Autodesk Inventor part; units mm, degrees
ref_plane "YZ Plane" through (0, 0, 0) normal (1, 0, 0) x (0, 1, 0)
ref_plane "XZ Plane" through (0, 0, 0) normal (0, 1, 0) x (-1, 0, 0)
ref_plane "XY Plane" through (0, 0, 0) normal (0, 0, 1) x (1, 0, 0)
sketch "Sketch1" plane through (0, 0, 0) normal (0, 0, 1) x (1, 0, 0)
  line L0 (0, 27.0856) -> (-1.414, 28.5)
  line L1 (-1.414, 28.5) -> (-1.414, 30)
  line L2 (-1.414, 30) -> (1.414, 30)
  line L3 (1.414, 30) -> (1.414, 28.5)
  line L4 (1.414, 28.5) -> (0, 27.0856)
  line L5 (-5, 0) -> (5, 0)
  point P0 (0, 0)
  point P1 (0, 30)
  point P2 (0, 0)
  dimension "d0" = 2
  dimension "d1" = 10
  dimension "d3" = 57
  dimension "d4" = 2.828
  dimension "d5" = 1.5
revolve "Revolution1" add sketch "Sketch1" angle 330 about axis through (-5, 0, 0) along (1, 0, 0)
properties part number "Pierścień klinowy"
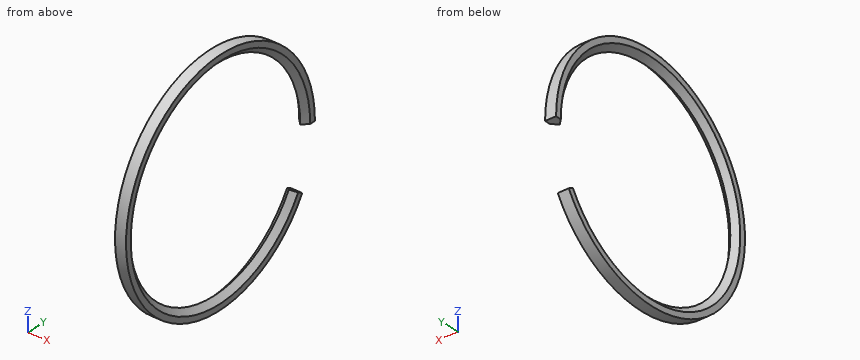
Source: CAD feature listing. Evaluate the final solid. Frame: model axes, mm. Round coordinates to 2 decimals unless told otherwise and drop trailing zeros. Loops run counter-clockwise (first coordinate to the right, second up) from the corner with the lowest first, then second, coordinate; pieces in that order, holes last. Notation, with made-up numbers: (63.25, 25.25) - (115.25, 25.25) arc R22 ccw to (115.25, 63.25) - close; hole circle Ø4 at (18, -26.5). An arc over 180 degrees is marked (long way). Write item = value, one per line. Start each with the question number.
(1) Pin query (flat end, axial travel): pin 1 (1 mm diameter, centred on x = 0, z = 15.5, fed in from -Y); pin 2 (1 mm diameter, centred on x = 1, y = 15.5, fed in from +Z); pin 3 (1.5 mm diameter, centred on x = -1, z = -21.5, fed in from +Y); pin 4 (8 mm diameter, centred on y = -0.5, z = -21.5, fed in from -X). Return the tip coordinate at first contact, or that it passes through.
(2) Ray query, line 1 along Z through (x, y) = (0.2, 1.5); line 2 along Y through (x, z) = (0.95, 10); line 3 along Y through (x, z) = (0.55, -22.5). Return the intervals inside material, ascending. Write a range as from..to.
(3) Section query A-A, the plane y = 0. Output: boundary loops of the cut face in (x, z), plus the area to 3 significant figures.
(4) Section query B-B, the plane x = -0.85. Output: boundary loops of the cut face in (y, z), plus the area to 3 significant figures.
Conclusion:
q1.pin_1 = -25.98
q1.pin_2 = 25.98
q1.pin_3 = 21.67
q1.pin_4 = through
q2.line_1 = -29.96..-27.24, 27.24..29.96
q2.line_2 = -28.28..-26.19, 26.19..28.28
q2.line_3 = -19.84..-16.05, 16.05..19.84
q3.outline = (-1.41, -30) - (1.41, -30) - (1.41, -28.5) - (0, -27.09) - (-1.41, -28.5) - close; (-1.41, 28.5) - (0, 27.09) - (1.41, 28.5) - (1.41, 30) - (-1.41, 30) - close
q3.area = 12.5 mm2
q4.outline = (24.19, -13.97) arc R27.94 cw (long way) to (27.94, 0) - (30, 0) arc R30 ccw (long way) to (25.98, -15) - close
q4.area = 344 mm2
